Geometry: final body of the model. Coordinates: model frame, mm. A direction names the side the tool comes from. Give positions to 0.01 mm unless a question says otherwise; leave off trailing zeros. Write each loop counter-clockwise with the first axis right and the second up, starting at its lowest first coordinate (ties: lowest second). Pieces come first, ordered by that corner, then holes. Notation, with made-up numbers: M 31.25,56 L 86.25,56 A17 ccw 86.25,85 Z; hole C -39,74.5 d1. An arc over 180 degrees is marked long. Use a Markdown table: item, result. Add a question column.
(1) Cut plane B-B (z = -5.5). Output: boundary loops of the cut face in (x, y) (1 decimal).
(2) Cut plane A-A (x = 73). Output: boundary loops of the cut face in (y, z).
(3) Reachability of faces 1 (the flat face through (-2, 0, -12.7)), 2 (the flat face through (-2, 11.112, 0)) from +Z, -Z, +X, -X, +Y, -Y: full face, straight path, thin tool, end or side. Return the list, or none.
(4) Material intervals for L1, parallel to Z at x = 45, y = 8.25, sorted ascending.
(5) Draft query along Y for faces 3 (the flat face through (-2, 12.7, 0)), 4 (the flat face through (-168.275, -11.3, 0.1)), 5 (the flat face through (-2, -12.7, 0)), 6 (the flat face through (-2, 0, 11.112)). Return one class per face: released by +Y, released by -Y, zero draft, split by the parting line, or undercut.
(6) Pin query (flat end, axial travel): pin 1 Ø2 at (y, z) = (-4.5, 10) entering from +X. Return the tip coordinate at first contact, or that it passes through.
Autodesk Inventor part; units mm, degrees
ref_plane "YZ Plane" through (0, 0, 0) normal (1, 0, 0) x (0, 1, 0)
ref_plane "XZ Plane" through (0, 0, 0) normal (0, 1, 0) x (-1, 0, 0)
ref_plane "XY Plane" through (0, 0, 0) normal (0, 0, 1) x (1, 0, 0)
sketch "Sketch1" plane through (0, 0, 0) normal (1, 0, 0) x (0, 1, 0)
  line L0 (-12.7, 12.7) -> (12.7, 12.7)
  line L1 (12.7, 12.7) -> (12.7, -12.7)
  line L2 (12.7, -12.7) -> (-12.7, -12.7)
  line L3 (-12.7, -12.7) -> (-12.7, 12.7)
  line L4 (-12.7, 12.7) -> (12.7, -12.7) construction
  line L5 (12.7, 12.7) -> (-12.7, -12.7) construction
  line L6 (-11.1125, 11.1125) -> (11.1125, 11.1125)
  line L7 (11.1125, 11.1125) -> (11.1125, -11.1125)
  line L8 (11.1125, -11.1125) -> (-11.1125, -11.1125)
  line L9 (-11.1125, -11.1125) -> (-11.1125, 11.1125)
  line L10 (-11.1125, 11.1125) -> (11.1125, -11.1125) construction
  line L11 (11.1125, 11.1125) -> (-11.1125, -11.1125) construction
  point P0 (0, 0)
  dimension "d0" = 25.4
  dimension "d1" = 1.5875
extrude "Extrusion1" add sketch "Sketch1" along normal mid plane 336.55
properties part number "cross brace" material "Aluminum 6061"
Answer list:
| question | item | result |
|---|---|---|
| 1 | outline | M -168.3,-12.7 L 168.3,-12.7 L 168.3,-11.1 L -168.3,-11.1 Z; M -168.3,11.1 L 168.3,11.1 L 168.3,12.7 L -168.3,12.7 Z |
| 2 | outline | M -12.7,-12.7 L 12.7,-12.7 L 12.7,12.7 L -12.7,12.7 Z; hole M -11.11,-11.11 L 11.11,-11.11 L 11.11,11.11 L -11.11,11.11 Z |
| 3 | face 1 | -Z, +X, -X, +Y, -Y |
| 3 | face 2 | +X, -X |
| 4 | L1 | -12.7 to -11.11, 11.11 to 12.7 |
| 5 | face 3 | released by +Y |
| 5 | face 4 | zero draft |
| 5 | face 5 | released by -Y |
| 5 | face 6 | undercut |
| 6 | pin 1 | through |
